Input: dimensioned drawing with shaded views. Units: mm. Origin: part minimum x, y, z. Coordinates: 2 decimals unless noted, no trailing zeros. Order: outer loops, then holes, each group sorted by start corner. A loop starts at its lowest first (then second) coordinate and runs counter-clockwise, first axis right, second up. Notation, with made-up numbers: (-4.5, 27) -> (10.5, 27) arc R26 ccw to (10.5, 55) -> close; hole circle Ø3 at (19, 70.5). An arc over 180 degrees is marked (long way). Answer as CSV lines item,"result".
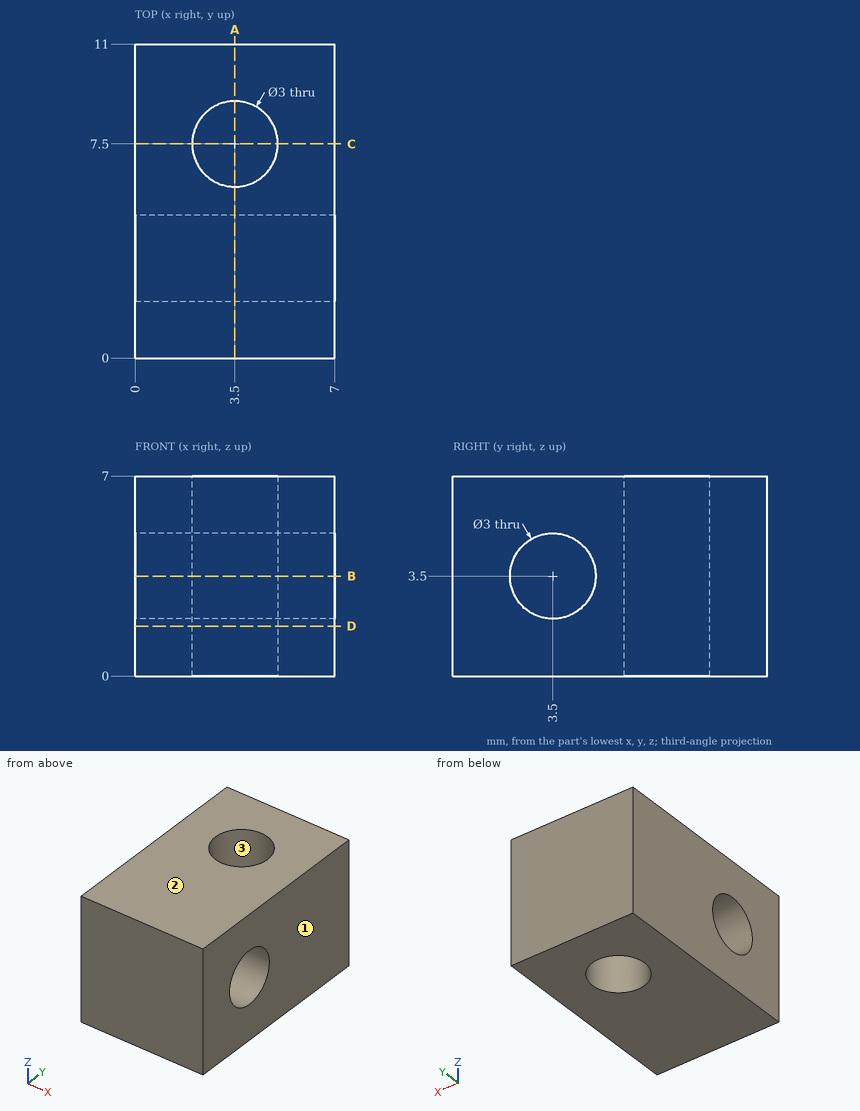
1. Cut plane B-B (z = 3.5). Return the cut outline in (x, y), plus the area to 3 significant figures.
Findings:
outline,"(0, 0) -> (7, 0) -> (7, 2) -> (0, 2) -> close; (0, 5) -> (7, 5) -> (7, 11) -> (0, 11) -> close; hole circle Ø3 at (3.5, 7.5)"
area,"48.9 mm2"
2. Ray query, line 1 along Z through (x, y) = (2.25, 3.5); line 2 along Y through (x, z) = (3.5, 2.5); line 3 along Y through (x, z) = (3.5, 4). Return the intervals inside material, ascending.
Findings:
line 1,"z = 0 to 2, 5 to 7"
line 2,"y = 0 to 2.38, 4.62 to 6, 9 to 11"
line 3,"y = 0 to 2.09, 4.91 to 6, 9 to 11"
3. Cut plane A-A (x = 3.5). Return the cut outline in (y, z), plus the area to 3 significant figures.
Findings:
outline,"(0, 0) -> (6, 0) -> (6, 7) -> (0, 7) -> close; (9, 0) -> (11, 0) -> (11, 7) -> (9, 7) -> close; hole circle Ø3 at (3.5, 3.5)"
area,"48.9 mm2"
4. Cut plane D-D (z = 1.75). Return the cut outline in (x, y), plus the area to 3 significant figures.
Findings:
outline,"(0, 0) -> (7, 0) -> (7, 11) -> (0, 11) -> close; hole circle Ø3 at (3.5, 7.5)"
area,"69.9 mm2"
5. Cut plane C-C (y = 7.5). Return the cut outline in (x, z), plus the area to 3 significant figures.
Findings:
outline,"(0, 0) -> (2, 0) -> (2, 7) -> (0, 7) -> close; (5, 0) -> (7, 0) -> (7, 7) -> (5, 7) -> close"
area,"28.0 mm2"
6. Mould query, pull axis X, two halves, no side actions, for the marked faces 1, 2 and 3. Classes: released by +X, released by -X, zero draft, split by the parting line, or undercut.
Findings:
face 1,"released by +X"
face 2,"zero draft"
face 3,"undercut"
